from build123d import *

# Parameters (mm, degrees)
SKETCH1_W                = 152.4
SKETCH1_H                = 31.75
BOSS_EXTRUDE1_DEPTH      = 6.35
BOSS_EXTRUDE2_DEPTH      = 12.7
BOSS_EXTRUDE2_DEPTH_BACK = 12.7
SKETCH7_R                = 9.525
BOSS_EXTRUDE4_DEPTH      = 12.7
BOSS_EXTRUDE5_REACH      = 250.235
BOSS_EXTRUDE5_END_RADIUS = 159.352919158
SKETCH8_W                = 17.78
SKETCH8_H                = 25.4


with BuildPart() as part:
    # Sketch1 → Boss-Extrude1 (new body)
    with BuildSketch(Plane(origin=(0, 0, 0), x_dir=(1, 0, 0), z_dir=(0, 1, 0))):
        with Locations((76.2, 15.875)):
            Rectangle(SKETCH1_W, SKETCH1_H)
    extrude(amount=BOSS_EXTRUDE1_DEPTH)

    # Sketch5 → Boss-Extrude2 (add, two sides)
    with BuildSketch(Plane(origin=(76.2, 0, 0), x_dir=(0, 0, -1), z_dir=(1, 0, 0))) as boss_extrude2_sk:
        with BuildLine():
            Line((6.218121971, 6.35), (25.531878029, 6.35))
            ThreePointArc((25.531878029, 6.35), (65.347005213, 88.504842335), (143.500563524, 135.69259281))
            Line((143.500563524, 135.69259281), (139.418467432, 151.35))
            ThreePointArc((139.418467432, 151.35), (51.469243862, 98.46173067), (6.218121971, 6.35))
        make_face()
    extrude(amount=BOSS_EXTRUDE2_DEPTH)
    extrude(boss_extrude2_sk.sketch, amount=-BOSS_EXTRUDE2_DEPTH_BACK)

    # Sketch7 → Boss-Extrude4 (add)
    with BuildSketch(Plane(origin=(0, 137.16, 0), x_dir=(1, 0, 0), z_dir=(0, 1, 0))):
        with Locations(Location((76.2, 130.81, 0), (0, 0, 270))):
            Circle(SKETCH7_R)
    extrude(amount=-BOSS_EXTRUDE4_DEPTH)

    # Boss-Extrude5: up to this cylinder (the profile starts outside it)
    boss_extrude5_end = Plane(origin=(76.2, -19.734844364, -184.022581395), z_dir=(1, 0, 0)) * Cylinder(BOSS_EXTRUDE5_END_RADIUS, 820.175838317, mode=Mode.PRIVATE)
    # Sketch8 → Boss-Extrude5 (add, up to the surface)
    with BuildSketch(Plane(origin=(0, 0, -19.05), x_dir=(-1, 0, 0), z_dir=(0, 0, -1)), mode=Mode.PRIVATE) as boss_extrude5_sk1:
        with Locations((-76.2, 25.4)):
            Rectangle(SKETCH8_W, SKETCH8_H)
    boss_extrude5_tool1 = extrude(boss_extrude5_sk1.sketch, amount=BOSS_EXTRUDE5_REACH, mode=Mode.PRIVATE) - boss_extrude5_end
    add(boss_extrude5_tool1.solids().sort_by_distance((76.2, 25.4, -19.05))[0])


solid = part.part
CAD build for the part. Positions are in the model's coordinates, mm. A direction names the side the tool comes from. Coordinates: 2 decimals unless noted, no trailing zeros. Write each loop counter-clockwise with the first axis right and the second up, starting at its lowest first coordinate (ties: lowest second). Pieces come first, ordered by that corner, then holes. Notation, with made-up numbers: (1, 27.5) - (35, 27.5) arc R10 cw to (35, 36.5) - close; hole circle Ø10 at (71.5, 74.25). An arc over 180 degrees is marked (long way). Use a Markdown table: item, result. Add a question column.
Item 1: Band-saw the part on D-D, the plane x = 27. Give the cut face in (y, z), and give its area (3 significant figures).
Item 2: Band-saw the part on C-C, the plane y = 17.5. Give the cut face in (x, z).
Item 3: Mould opens along Y. For faces 6 (the face through (76.38, 143.41, -141.49)), 7 (the face through (88.9, 85, -59)), 8 (the face through (75, 0, -16)), 9 (the face through (85.09, 25, -30)) say: pulls with the +Y half, pulls with the -Y half, needs draft (parallel to the pull), parting line crosses it, or undercut.
Item 4: Flat gauge pins, fed straight in: pin 1 (0.7 mm diameter, centred on x = 79.5, z = -35, fed in from +Y); pin 2 (5 mm diameter, centred on x = 66.5, y = 49, fed in from -Z); pin 3 (4.5 mm diameter, centred on y = 27, z = -31.5, fed in from -X); pin 4 (1 mm diameter, centred on x = 77.5, z = -27, fed in from -Y). Where does each tip first touch, or does it go through?
Item 5: 3-axis set-ups, long thin cutter, end or side, ignore diameter. For faces 1 (the face through (152.4, 3, -16)), 2 (the face through (76.324, 25.735, -31.294)), 3 (the face through (63.5, 85, -59)), 4 (the face through (76, 124.46, -131)), 5 (the face through (76.02, 99.53, -52.46)): which of +Z, -Z, +X, -X, +Y, -Y reach the whole face in a straight line?
Item 6: Band-saw the part on A-A, the plane x = 76.2. Give the cut face in (y, z) (3 decimals).
Item 7: Band-saw the part on B-B, the plane z = -127.5. Give the cut face in (x, y), and give its area (3 significant figures).
Item 8: Drill centre lines: L1, parallel to X at y = 41, z = -30; L2, parallel to Y at x = 26, z = -7.5; L3, parallel to Z at x = 81.5, y = 129. Where is each one in solid material? Low to high. Write a range as from..to.
Numbers:
| question | item | result |
|---|---|---|
| 1 | outline | (0, -31.75) - (6.35, -31.75) - (6.35, 0) - (0, 0) - close |
| 1 | area | 202 mm2 |
| 2 | outline | (63.5, -27.78) - (67.31, -27.78) - (67.31, -29.08) - (85.09, -29.08) - (85.09, -27.78) - (88.9, -27.78) - (88.9, -8.5) - (63.5, -8.5) - close |
| 3 | face 6 | pulls with the +Y half |
| 3 | face 7 | needs draft |
| 3 | face 8 | pulls with the -Y half |
| 3 | face 9 | undercut |
| 4 | pin 1 | y = 78.18 |
| 4 | pin 2 | z = -40.06 |
| 4 | pin 3 | x = 63.5 |
| 4 | pin 4 | y = 0 |
| 5 | face 1 | +Z, -Z, +X, +Y, -Y |
| 5 | face 2 | -Z, +X, -X |
| 5 | face 3 | +Z, -Z, -X, +Y |
| 5 | face 4 | -Z, +X, -X, -Y |
| 5 | face 5 | +Z, +X, -X, +Y |
| 6 | outline | (0, -31.75) - (6.35, -31.75) - (6.35, -25.532) arc R160.623 cw to (12.7, -26.709) - (12.7, -28.005) arc R159.353 cw to (38.1, -35.535) - (38.1, -34.173) arc R160.623 cw to (128.129, -121.285) - (124.46, -121.285) - (124.46, -140.335) - (134.833, -140.335) arc R160.623 cw to (135.693, -143.501) - (151.35, -139.418) arc R181.655 ccw to (6.35, -6.218) - (6.35, 0) - (0, 0) - close |
| 7 | outline | (63.5, 130.61) - (67.27, 130.61) - (67.27, 124.46) - (85.13, 124.46) - (85.13, 130.61) - (88.9, 130.61) - (88.9, 147.8) - (63.5, 147.8) - close |
| 7 | area | 547 mm2 |
| 8 | L1 | 63.5..88.9 |
| 8 | L2 | 0..6.35 |
| 8 | L3 | -138.72..-87.99 |
